Verification items for the finished model (mm, model axes). Round coordinates to 2 decimals unless told otherwise and drop trailing zeros. Write each loop counter-clockwise with the first axis right and the second up, starting at its lowest first coordinate (ties: lowest second). Pieces come first, ordered by that corner, then holes. Notation, with made-up numbers: M 82,1 L 105,1 A24 cw 105,36 Z; hole C -14,-26 d7. An arc over 180 degrees is marked long. One line per question, with ' | ' between items.
from build123d import *

# Parameters (mm, degrees)
F0_R     = 1
F0_R_2   = 1.6
F1_DEPTH = 4


# Not quite as in the source:
# - a feature names something its author has since deleted; it is built from what else it names


with BuildPart() as f1:
    # F0 (on Top) → F1 (new body)
    with BuildSketch(Plane.XY):
        Polygon((-69.85, 0), (-69.85, -8.5), (15.9242544323, -8.5), (69.85, -2.218887916), (69.85, 8.5), (-15.9242544323, 8.5), align=None)
        with Locations((-5.6605379174, -5.6497372861)):
            Circle(F0_R, mode=Mode.SUBTRACT)
        with Locations((4.2389570192, -4.2355237237)):
            Circle(F0_R, mode=Mode.SUBTRACT)
        with Locations((-4.2463243551, 4.2497576505)):
            Circle(F0_R, mode=Mode.SUBTRACT)
        Circle(F0_R_2, mode=Mode.SUBTRACT)
        with Locations((5.6531705815, 5.6639712129)):
            Circle(F0_R, mode=Mode.SUBTRACT)
    extrude(amount=F1_DEPTH)


solid = f1.part
1. Mould release check, pull along X, two halves, no side actions. Record for faces 1 (the face through (-1, -2, 0)), 2 (the face through (-42.51, 4.31, 1.97)), 3 (the face through (-1.27, -0.97, 1.97)): pulls with the +X half, pulls with the -X half, needs draft (parallel to the pull), parting line crosses it, or undercut.
Results:
face 1: needs draft | face 2: pulls with the -X half | face 3: undercut
2. Section check D-D, the plane x = 20. Record the cut outline in (y, z).
Results:
outline: M -8.03,0 L 8.5,0 L 8.5,4 L -8.03,4 Z
3. Section check C-C, the plane x = -36. Record the cut outline in (y, z).
Results:
outline: M -8.5,0 L 5.34,0 L 5.34,4 L -8.5,4 Z
4. Section check B-B, the plane z = 2.4. Record the cut outline in (x, y), then the cut area to 3 significant figures.
Results:
outline: M -69.85,-8.5 L 15.92,-8.5 L 69.85,-2.22 L 69.85,8.5 L -15.92,8.5 L -69.85,0 Z; hole C -5.66,-5.65 d2; hole C -4.25,4.25 d2; hole C 0,0 d3.2; hole C 4.24,-4.24 d2; hole C 5.65,5.66 d2 | area: 1,960 mm2
5. Thickness scan on line 1 (X direction, y = -0.25, z = 3.85); line 2 (Y direction, x = -27.5, z = 1.5); line 3 (Y direction, x = 39.5, z = 3.1). Record the ranges inside material, lowest first.
Results:
line 1: x = -69.85 to -1.58, 1.58 to 69.85 | line 2: y = -8.5 to 6.68 | line 3: y = -5.75 to 8.5
6. Section check A-A, the plane x = 0. Record the cut outline in (y, z).
Results:
outline: M -8.5,0 L -1.6,0 L -1.6,4 L -8.5,4 Z; M 1.6,0 L 8.5,0 L 8.5,4 L 1.6,4 Z
